Autodesk Inventor part; units mm, degrees
ref_plane "YZ Plane" through (0, 0, 0) normal (1, 0, 0) x (0, 1, 0)
ref_plane "XZ Plane" through (0, 0, 0) normal (0, 1, 0) x (-1, 0, 0)
ref_plane "XY Plane" through (0, 0, 0) normal (0, 0, 1) x (1, 0, 0)
sketch "Sketch1" plane through (0, 0, 0) normal (0, 1, 0) x (-1, 0, 0)
  circle A0 centre (0, 0) radius 31.75 construction
  circle A1 centre (0, -63.5) radius 31.75 construction
  circle A2 centre (0, 0) radius 9.525
  circle A3 centre (0, -63.5) radius 9.525
  circle A4 centre (0, 0) radius 25.4 construction
  circle A5 centre (0, -63.5) radius 25.4 construction
  circle A6 centre (0, 25.4) radius 2.4892
  circle A7 centre (-21.997, 12.7) radius 2.4892
  circle A8 centre (-21.997, -12.7) radius 2.4892
  circle A9 centre (0, -25.4) radius 2.4892
  circle A10 centre (21.997, -12.7) radius 2.4892
  circle A11 centre (21.997, 12.7) radius 2.4892
  circle A12 centre (0, -88.9) radius 2.4892
  circle A13 centre (21.997, -76.2) radius 2.4892
  circle A14 centre (21.997, -50.8) radius 2.4892
  circle A15 centre (0, -38.1) radius 2.4892
  circle A16 centre (-21.997, -50.8) radius 2.4892
  circle A17 centre (-21.997, -76.2) radius 2.4892
  circle A18 centre (-32.9859, -31.75) radius 36.2585 construction
  circle A19 centre (-32.9859, -31.75) radius 14.2875
  circle A20 centre (0, -63.5) radius 44.45
  circle A21 centre (0, 0) radius 44.45
  circle A22 centre (-32.9859, -31.75) radius 48.9585
  circle A23 centre (-39.4239, 14.2199) radius 2.4892
  circle A24 centre (-39.4239, 14.2199) radius 6.35 construction
  line L0 (-29.8666, 10.7726) -> (-33.4506, 12.0653) construction
  line L1 (-38.5432, 7.9312) -> (-38.0147, 4.1581) construction
  circle A25 centre (-39.4239, -77.7199) radius 2.4892
  circle A26 centre (-39.4239, -77.7199) radius 6.35 construction
  line L2 (-33.4506, -75.5653) -> (-29.8666, -74.2726) construction
  line L3 (-38.5432, -71.4312) -> (-38.0147, -67.6581) construction
  circle A27 centre (27.3566, -31.75) radius 2.4892
  circle A28 centre (27.3566, -31.75) radius 6.35 construction
  line L4 (23.2117, -26.9394) -> (20.7247, -24.053) construction
  line L5 (23.2117, -36.5606) -> (20.7247, -39.447) construction
  line L6 (44.45, 0) -> (44.45, -63.5)
  line L7 (-27.5218, 34.9049) -> (-63.2991, 6.6953)
  line L8 (-63.2991, -70.1953) -> (-27.5218, -98.4049)
  circle A29 centre (-75.5944, -31.75) radius 6.35 construction
  circle A30 centre (-75.5944, -31.75) radius 2.4892
  point P0 (31.1085, -31.75)
  dimension "d4" = 50.8
  dimension "d0" = 63.5
  dimension "d2" = 19.05
  dimension "d5" = 4.9784
  dimension "d8" = 360
  dimension "d12" = 360
  dimension "d14" = 72.517
  dimension "d15" = 28.575
  dimension "d38" = 45.7835
  dimension "d39" = 12.7
  dimension "d40" = 12.7
  dimension "d41" = 12.7
  dimension "d42" = 4.9784
  dimension "d43" = 12.7
  dimension "d44" = 3.81
extrude "Extrusion2" add sketch "Sketch1" along normal blind 3.175 contours A2 A22 A21 A20 | A2 A22 A20 A19 A21 | A22 L7 A21 | A21 A19 A20 A22 | A22 A21 A19 A20 | A20 A21 A22 | A21 L6 A20 | A20 A22 A3 A21 | A19 A21 A22 A3 A20 | A22 A20 L8
properties part number "Gearboxes_3_thingy that holds motors and more" material "Aluminum 6061"
Part model, mm, in its own coordinate system. Coordinates: 2 decimals unless noted, no trailing zeros. Order: outer loops, then holes, each group sorted by start corner. A loop starts at its lowest first (then second) coordinate and runs counter-clockwise, first axis right, second up. Notation, with made-up numbers: (76.25, 49.5) - (131.25, 49.5) arc R26 cw to (131.25, 78.5) - close; hole circle Ø5 at (22, -0.75). An arc over 180 degrees is marked (long way). Return JSON: item names as keys, results as strings. Group by question number.
Item 1: Pin check, flat tips, straight feed: pin 1 (4.5 mm diameter, centred on x = -21.997, z = -76.2, fed in from -Y); pin 2 (22 mm diameter, centred on x = 0, z = -63.5, fed in from -Y); pin 3 (1.5 mm diameter, centred on x = 44, y = 2, fed in from -Z). Stop position of each tip, or through.
Item 2: Cut at D-D (z = -12.7). List the corners of the cut face in (x, y) (3 decimals), plus the area to 3 significant figures.
Item 3: Cut at A-A (z = -31.75). List the corners of the cut face in (x, y) (3 decimals), plus the area to 3 significant figures.
Item 4: Pull direction Z, two halves, no side cores. Call faces 1 (the face through (6, 3.175, -31)), 2 (the face through (-18.768, 1.565, 40.294)), 3 (the face through (22.32, 1.57, -15.17)): pulls with the +Z half, pulls with the -Z half, needs draft (parallel to the pull), parting line crosses it, or undercut.
Item 5: Cut at B-B (z = -88.9). List the corners of the cut face in (x, y) (3 decimals).
Item 6: Drill centre lines: probe 1 along Z at (x, y) = (-24, 2.85); probe 2 along Z at (x, y) = (4.5, 2.4); probe 3 along X at (y, z) = (1.1, -50). Where is each one in solid material? Low to high. Write a range as from..to.
Item 7: Cut at C-C (y = 2.3). State how many separate pieces and enclosed holes the cut face has, plus the area to 3 significant figures.
Check values:
{
 "1": {"pin 1": "passes through", "pin 2": "stops at y = 0", "pin 3": "stops at z = -86"},
 "2": {"outline": "(-44.45, 0) - (-24.486, 0) - (-24.486, 3.175) - (-44.45, 3.175) - close; (-19.508, 0) - (19.508, 0) - (19.508, 3.175) - (-19.508, 3.175) - close; (24.486, 0) - (78.086, 0) - (78.086, 3.175) - (24.486, 3.175) - close", "area": "357 mm2"},
 "3": {"outline": "(-44.45, 0) - (-29.846, 0) - (-29.846, 3.175) - (-44.45, 3.175) - close; (-24.867, 0) - (18.698, 0) - (18.698, 3.175) - (-24.867, 3.175) - close; (47.273, 0) - (73.105, 0) - (73.105, 3.175) - (47.273, 3.175) - close; (78.084, 0) - (81.944, 0) - (81.944, 3.175) - (78.084, 3.175) - close", "area": "279 mm2"},
 "4": {"face 1": "needs draft", "face 2": "pulls with the +Z half", "face 3": "undercut"},
 "5": {"outline": "(-36.478, 0) - (-2.489, 0) - (-2.489, 3.175) - (-36.478, 3.175) - close; (2.489, 0) - (39.577, 0) - (39.577, 3.175) - (2.489, 3.175) - close"},
 "6": {"probe 1": "z = -100.91..-77.68, -74.72..-52.28, -49.32..-14.18, -11.22..11.22, 14.18..37.41", "probe 2": "z = -107.72..-71.89, -55.11..-8.39, 8.39..44.22", "probe 3": "x = -44.45..-24.35, -19.64..19.64, 24.35..78.42"},
 "7": {"separate pieces": "1", "enclosed holes": "19", "area": "13,200 mm2"}
}
